The model under review builds one solid part; all positions refer to its coordinate system, in mm. Face numbers are marked on the shaded views. A direction names the side the tool comes from. Round coordinates to 2 decimals unless told otherwise and drop trailing zeros. Order: outer loops, then holes, each group sorted by start corner. A loop starts at its lowest first (then second) coordinate and runs counter-clockwise, first axis right, second up.
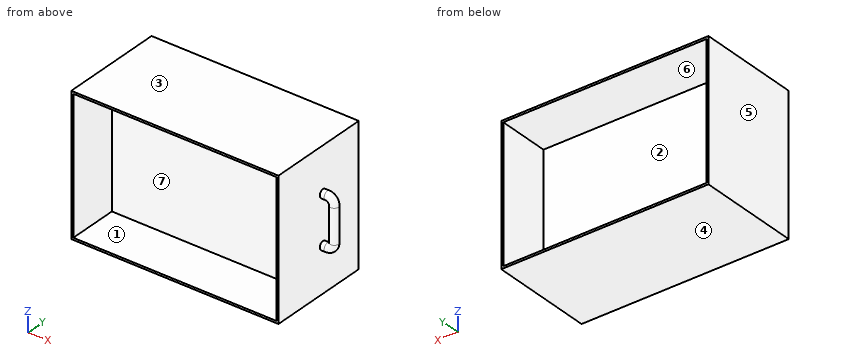
```python
from build123d import *

# Parameters (mm, degrees)
SKETCH1_W                 = 300
SKETCH1_H                 = 200
BOSS_EXTRUDE1_DEPTH       = 150
SHELL1_T                  = -3
SHELL1_THICKNESS_2_FACE_W = 194
SHELL1_THICKNESS_2_FACE_H = 294
SHELL1_THICKNESS_2_DEPTH  = 72
SHELL2_START              = -133.820083682
SHELL2_OUTLINE_W          = 72
SHELL2_OUTLINE_H          = 194
SHELL2_DEPTH              = 294
SKETCH2_R                 = 6


# Read off the part's stored shape, not the designer's step: Shell2
with BuildPart() as part:
    # Sketch1 → Boss-Extrude1 (new body)
    with BuildSketch(Plane(origin=(0, 0, 0), x_dir=(1, 0, 0), z_dir=(0, 1, 0))):
        with Locations((13.179916318, 19.874476987)):
            Rectangle(SKETCH1_W, SKETCH1_H)
    extrude(amount=BOSS_EXTRUDE1_DEPTH)

    # Shell1
    shell1_openings = [part.faces().sort_by_distance(p)[0] for p in [
        (13.179916318, 150, -19.874476987),
    ]]
    offset(amount=SHELL1_T, openings=shell1_openings, kind=Kind.INTERSECTION)

    # Shell1 thickness 2 face (on inner face of the shell) → Shell1 thickness 2 (add)
    with BuildSketch(Plane(origin=(13.179916318, 3, -19.874476987), x_dir=(0, 0, -1), z_dir=(0, -1, 0))):
        Rectangle(SHELL1_THICKNESS_2_FACE_W, SHELL1_THICKNESS_2_FACE_H)
    extrude(amount=-SHELL1_THICKNESS_2_DEPTH)

    # Shell2 outline → Shell2 (cut)
    with BuildSketch(Plane.YZ.offset(SHELL2_START)):
        with Locations((36, -19.874476987)):
            Rectangle(SHELL2_OUTLINE_W, SHELL2_OUTLINE_H)
    extrude(amount=SHELL2_DEPTH, mode=Mode.SUBTRACT)

    # Sweep2: sweep along a path in Sketch4
    with BuildLine(Plane(origin=(0, 83.172395684, 0), x_dir=(1, 0, 0), z_dir=(0, 1, 0))) as sweep2_path:
        Line((163.179916318, -15.125523013), (169.565605174, -15.125523013))
        ThreePointArc((169.565605174, -15.125523013), (176.636672985, -12.196590824), (179.565605174, -5.125523013))
        Line((179.565605174, -5.125523013), (179.565605174, 44.874476987))
        ThreePointArc((179.565605174, 44.874476987), (176.636672985, 51.945544799), (169.565605174, 54.874476987))
        Line((169.565605174, 54.874476987), (163.179916318, 54.874476987))
    # Sketch2 → Sweep2 (sweep)
    with BuildSketch(Plane(origin=(163.179916318, 0, 0), x_dir=(0, 0, -1), z_dir=(1, 0, 0))):
        with Locations((-15.125523013, 83.172395684)):
            Circle(SKETCH2_R)
    sweep(path=sweep2_path.line)


solid = part.part
```
(1) Consider section B-B (x = 13.5). Write out the cut boundary in (y, z).
Data:
outline: (0, -119.87) - (150, -119.87) - (150, -116.87) - (75, -116.87) - (75, 77.13) - (150, 77.13) - (150, 80.13) - (0, 80.13) - (0, 77.13) - (72, 77.13) - (72, -116.87) - (0, -116.87) - close
(2) Consider section C-C (z = 64). Write out the cut boundary in (x, y), and give its area (3 significant figures).
Data:
outline: (-136.82, 0) - (-133.82, 0) - (-133.82, 72) - (160.18, 72) - (160.18, 0) - (163.18, 0) - (163.18, 150) - (160.18, 150) - (160.18, 75) - (-133.82, 75) - (-133.82, 150) - (-136.82, 150) - close
area: 1,780 mm2
(3) For the marked faces 1, 2 and 3, list the 3-axis set-ups (+Z, -Z, +X, -X, +Y, -Y) from which the entire face can be reached by the end or side of a thin tool; tool diameter is ignored.
Data:
face 1: -Y
face 2: +Y
face 3: +Z, +X, -X, +Y, -Y
(4) To check wall thickness, follow probe 1 along Z at (x, y) = (128, 118.5); probe 2 along X at (y, z) = (102, -100); probe 3 along X at (y, z) = (79, -21). State the ranges of each line that lie inside material, in increasing order.
Data:
probe 1: z = -119.87 to -116.87, 77.13 to 80.13
probe 2: x = -136.82 to -133.82, 160.18 to 163.18
probe 3: x = -136.82 to -133.82, 160.18 to 163.18, 175.25 to 183.88
(5) Draft analysis for pull direction Z (two halves, no side actions). For the marked faces 4, 5, 6 and 7, state which applies: pulls with the +Z half, pulls with the -Z half, needs draft (parallel to the pull), parting line crosses it, or undercut.
Data:
face 4: pulls with the -Z half
face 5: needs draft
face 6: undercut
face 7: undercut
(6) Consider section D-D (z = -25). Write out the cut boundary in (x, y), and give its area (3 significant figures).
Data:
outline: (-136.82, 0) - (-133.82, 0) - (-133.82, 72) - (160.18, 72) - (160.18, 0) - (163.18, 0) - (163.18, 150) - (160.18, 150) - (160.18, 75) - (-133.82, 75) - (-133.82, 150) - (-136.82, 150) - close; circle Ø12 at (179.57, 83.17)
area: 1,900 mm2
(7) Insertion check: pin 1 (1.5 mm diameter, centred on y = 38, z = -86, fed in from +X); pin 2 (1.5 mm diameter, centred on x = -25, z = -38.5, fed in from +Y); pin 3 (5 mm diameter, centred on x = 80, z = -79.5, fed in from -Y). Each pin has a flat end and moves straight along its axis. Give the tip position at first contact, or say it passes through.
Data:
pin 1: stops at x = 163.18
pin 2: stops at y = 75
pin 3: stops at y = 72
(8) Consider section A-A (y = 10.5). Write out the cut boundary in (x, z).
Data:
outline: (-136.82, -119.87) - (163.18, -119.87) - (163.18, 80.13) - (-136.82, 80.13) - close; hole (-133.82, -116.87) - (160.18, -116.87) - (160.18, 77.13) - (-133.82, 77.13) - close
